The listing builds one solid part. Answer for the finished solid, in the listing's coordinates (mm). A direction names the side the tool comes from. Round coordinates to 2 decimals unless told otherwise and drop trailing zeros. Write each loop counter-clockwise with the first axis right and the second up, starting at its lowest first coordinate (ties: lowest second). Pieces come first, ordered by that corner, then holes.
from build123d import *

# Parameters (mm, degrees)
F1_DEPTH  = 30
F2_R      = 4.25
F3_DEPTH  = 5
F5_R      = 4.25
F5_R_2    = 3.75
F6_DEPTH  = 3
F7_R      = 1.075
F8_DEPTH  = 5
F9_R      = 3
F10_DEPTH = 1.1


with BuildPart() as f1:
    # F0 (on Top) → F1 (new body)
    with BuildSketch(Plane.XY):
        Polygon((-2.5, -1.0355339059), (-2.5, -2.5), (-1.0355339059, -2.5), align=None)
        Polygon((-2.5, -1.0355339059), (-1.0355339059, -2.5), (1.0355339059, -2.5), (2.5, -1.0355339059), (2.5, 1.0355339059), (1.0355339059, 2.5), (-1.0355339059, 2.5), (-2.5, 1.0355339059), align=None)
        Polygon((1.0355339059, -2.5), (-1.0355339059, -2.5), (0, -3.5355339059), align=None)
        Polygon((-3.5355339059, 0), (-2.5, -1.0355339059), (-2.5, 1.0355339059), align=None)
        Polygon((2.5, -1.0355339059), (1.0355339059, -2.5), (2.5, -2.5), align=None)
        Polygon((-2.5, 2.5), (-2.5, 1.0355339059), (-1.0355339059, 2.5), align=None)
        Polygon((2.5, 1.0355339059), (2.5, -1.0355339059), (3.5355339059, 0), align=None)
        Polygon((0, 3.5355339059), (-1.0355339059, 2.5), (1.0355339059, 2.5), align=None)
        Polygon((1.0355339059, 2.5), (2.5, 1.0355339059), (2.5, 2.5), align=None)
    extrude(amount=F1_DEPTH)

    # F2 (on face) → F3 (join)
    with BuildSketch(Plane(origin=(0, 0, 0), x_dir=(1, 0, 0), z_dir=(0, 0, -1))):
        Circle(F2_R)
    extrude(amount=F3_DEPTH)

    # F5 (on offset) → F6 (cut)
    with BuildSketch(Plane(origin=(0, 0, -4), x_dir=(1, 0, 0), z_dir=(0, 0, -1))):
        Circle(F5_R)
        Circle(F5_R_2, mode=Mode.SUBTRACT)
    extrude(amount=-F6_DEPTH, mode=Mode.SUBTRACT)

    # F7 (on Top) → F8 (cut)
    with BuildSketch(Plane.XY):
        Circle(F7_R)
    extrude(amount=-F8_DEPTH, mode=Mode.SUBTRACT)

    # F9 (on face) → F10 (cut)
    with BuildSketch(Plane(origin=(0, 0, -5), x_dir=(1, 0, 0), z_dir=(0, 0, -1))):
        Circle(F9_R)
    extrude(amount=-F10_DEPTH, mode=Mode.SUBTRACT)


solid = f1.part
1. Section C-C on x = 2 is taken. Determine the outline of the cut face in (y, z).
Geometry says:
outline: (-3.75, -5) - (-2.24, -5) - (-2.24, -3.9) - (2.24, -3.9) - (2.24, -5) - (3.75, -5) - (3.75, -4) - (3.17, -4) - (3.17, -1) - (3.75, -1) - (3.75, 0) - (2.5, 0) - (2.5, 30) - (-2.5, 30) - (-2.5, 0) - (-3.75, 0) - (-3.75, -1) - (-3.17, -1) - (-3.17, -4) - (-3.75, -4) - close
2. Given pin 1 (0.7 mm diameter, centred on x = 2, z = 14, fed in from +Y); pin 2 (1.6 mm diameter, centred on y = 1.5, z = 11, fed in from -X); pin 3 (5 mm diameter, centred on y = 3.5, z = 10, fed in from +X); pin 4 (3 mm diameter, centred on x = -1.5, y = -1, fed in from -Z), each flat-ended and moving along its own axis, determine where each tip first touches the part or whether it passes through.
Geometry says:
pin 1: stops at y = 2.5
pin 2: stops at x = -2.84
pin 3: stops at x = 2.54
pin 4: stops at z = -5
3. Section A-A on z = 14 is taken. Determine the outline of the cut face in (x, y), plus the area to 3 significant figures.
Geometry says:
outline: (-3.54, 0) - (-2.5, -1.04) - (-2.5, -2.5) - (-1.04, -2.5) - (0, -3.54) - (1.04, -2.5) - (2.5, -2.5) - (2.5, -1.04) - (3.54, 0) - (2.5, 1.04) - (2.5, 2.5) - (1.04, 2.5) - (0, 3.54) - (-1.04, 2.5) - (-2.5, 2.5) - (-2.5, 1.04) - close
area: 29.3 mm2
4. Straight lines are drawn through the part: line 1 along Y through (x, z) = (0, -2.5) (3 decimals); line 2 along X through (y, z) = (0, -4.45); line 3 along X through (y, z) = (-1.25, 7). For each, find the intervals that lie inside material, in ascending order.
Geometry says:
line 1: y = -3.75 to -1.075, 1.075 to 3.75
line 2: x = -4.25 to -3, 3 to 4.25
line 3: x = -2.5 to 2.5
5. For a pull along Z with two mould halves and no side action, classify faces 1 (the face through (-2, 2.5, 15)), 2 (the face through (0, 0, 0)), 3 (the face through (0, 4, -1)) as released by +Z, released by -Z, zero draft, split by the parting line, or undercut.
Geometry says:
face 1: zero draft
face 2: released by -Z
face 3: undercut
6. Section B-B on y = -1.5 is taken. Determine the outline of the cut face in (x, z).
Geometry says:
outline: (-3.98, -5) - (-2.6, -5) - (-2.6, -3.9) - (2.6, -3.9) - (2.6, -5) - (3.98, -5) - (3.98, -4) - (3.44, -4) - (3.44, -1) - (3.98, -1) - (3.98, 0) - (2.5, 0) - (2.5, 30) - (-2.5, 30) - (-2.5, 0) - (-3.98, 0) - (-3.98, -1) - (-3.44, -1) - (-3.44, -4) - (-3.98, -4) - close
7. Section D-D on x = -0.5 is taken. Determine the outline of the cut face in (y, z), plus the area to 3 significant figures.
Geometry says:
outline: (-4.22, -5) - (-2.96, -5) - (-2.96, -3.9) - (-0.95, -3.9) - (-0.95, 0) - (0.95, 0) - (0.95, -3.9) - (2.96, -3.9) - (2.96, -5) - (4.22, -5) - (4.22, -4) - (3.72, -4) - (3.72, -1) - (4.22, -1) - (4.22, 0) - (3.04, 0) - (3.04, 30) - (-3.04, 30) - (-3.04, 0) - (-4.22, 0) - (-4.22, -1) - (-3.72, -1) - (-3.72, -4) - (-4.22, -4) - close
area: 207 mm2
8. A tool of negligible diameter and unlimited length cuts with its end or side. For faces 4 (the face through (0.525, 3.011, 14.79)), 5 (the face through (0.511, -3.025, 14.79)), 6 (the face through (-2, -2.5, 15)), from which of +Z, -Z, +X, -X, +Y, -Y can it reach the whole face along a straight path? Write none if from no direction.
Geometry says:
face 4: +Z, +X, +Y
face 5: +Z, +X, -Y
face 6: +Z, -X, -Y
